```python
from build123d import *

# Parameters (mm, degrees)
SKETCH1_R             = 3.5
BOSS_EXTRUDE1_DEPTH   = 4
SKETCH2_R             = 1.925
BOSS_EXTRUDE2_DEPTH   = 10
CUT_EXTRUDE1_DEPTH    = 2
CHAMFER1_SIZE         = 0.25
CHAMFER1_SIZE2        = 0.209774908
CHAMFER1_PART_2_SIZE  = 0.25
CHAMFER1_PART_2_SIZE2 = 0.209774908
CHAMFER1_PART_3_SIZE  = 0.25
CHAMFER1_PART_3_SIZE2 = 0.209774908


with BuildPart() as part:
    # Sketch1 → Boss-Extrude1 (new body)
    with BuildSketch(Plane(origin=(0, 0, 0), x_dir=(1, 0, 0), z_dir=(0, 1, 0))):
        Circle(SKETCH1_R)
    extrude(amount=BOSS_EXTRUDE1_DEPTH)

    # Sketch2 → Boss-Extrude2 (add)
    with BuildSketch(Plane(origin=(0, 4, 0), x_dir=(1, 0, 0), z_dir=(0, 1, 0))):
        Circle(SKETCH2_R)
    extrude(amount=BOSS_EXTRUDE2_DEPTH)

    # Sketch3 → Cut-Extrude1 (cut)
    with BuildSketch(Plane.XZ):
        Polygon((0, 2.37190351), (-2.054128695, 1.185951755), (-2.054128695, -1.185951755), (0, -2.37190351), (2.054128695, -1.185951755), (2.054128695, 1.185951755), align=None)
    extrude(amount=-CUT_EXTRUDE1_DEPTH, mode=Mode.SUBTRACT)

    # Chamfer1
    chamfer1_edges = [part.edges().sort_by_distance(p)[0] for p in [
        (1.027064348, 0, 1.778927633),
        (-1.027064348, 0, 1.778927633),
        (-2.054128695, 0, 0),
        (-1.027064348, 0, -1.778927633),
        (1.027064348, 0, -1.778927633),
        (2.054128695, 0, 0),
        (-3.5, 0, 0),
    ]]
    chamfer1_side = [part.faces().sort_by_distance(p)[0] for p in [
        (-3.401005051, 0, 0),
    ]]
    chamfer(chamfer1_edges, length=CHAMFER1_SIZE, length2=CHAMFER1_SIZE2, reference=chamfer1_side[0])

    # Chamfer1 part 2
    chamfer1_part_2_edges = [part.edges().sort_by_distance(p)[0] for p in [
        (-3.5, 4, 0),
    ]]
    chamfer1_part_2_side = [part.faces().sort_by_distance(p)[0] for p in [
        (-3.5, 2, 0),
    ]]
    chamfer(chamfer1_part_2_edges, length=CHAMFER1_PART_2_SIZE, length2=CHAMFER1_PART_2_SIZE2, reference=chamfer1_part_2_side[0])

    # Chamfer1 part 3
    chamfer1_part_3_edges = [part.edges().sort_by_distance(p)[0] for p in [
        (-1.925, 14, 0),
    ]]
    chamfer1_part_3_side = [part.faces().sort_by_distance(p)[0] for p in [
        (-1.925, 9, 0),
    ]]
    chamfer(chamfer1_part_3_edges, length=CHAMFER1_PART_3_SIZE, length2=CHAMFER1_PART_3_SIZE2, reference=chamfer1_part_3_side[0])


solid = part.part
```
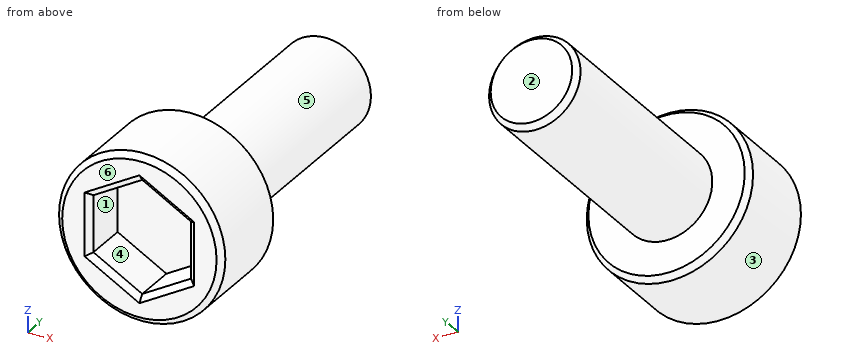
Can you work these out from the model? Positions are in its coordinate system, mm. Face numbers are marked on the shaded views. A direction names the side the tool comes from. Round coordinates to 2 decimals unless told otherwise and drop trailing zeros. Loops run counter-clockwise (first coordinate to the right, second up) from the corner with the lowest first, then second, coordinate; pieces in that order, holes last. Notation, with made-up numbers: M 13,-9 L 61,-9 A10 cw 61,5 Z; hole C 88,60 d6. An arc over 180 degrees is marked long. Answer as a JSON object with one key per item and string values. Group by question number.
Q1. Imagine slicing it at C-C, the plane y = 10.25. Please give me the cut outline in (x, z) (3 decimals), then the cut area to 3 significant figures.
Q2. Imagine slicing it at A-A, the plane z = 0. Please give me the cut outline in (x, y) (3 decimals), then the cut area to 3 significant figures.
Q3. Imagine slicing it at B-B, the plane y = 3.5. Please give me the cut outline in (x, z), then the cut area to 3 significant figures.
Q4. Please list where these lines run through material, in increasing order: L1, parallel to Y at x = -0.5, z = 0; L2, parallel to Y at x = -1, z = -3; L3, parallel to X at y = 1.5, z = 2.25.
Q5. On a 3-axis mill with a long thin cutter (end or side, diameter ignored), from which of +Z, -Z, +X, -X, +Y, -Y can I reach the whole of each face in a straight line? I mean the marked faces 4, 5 and 6. Say none if no direction works.
Q6. We'd pull the mould along X, two halves only. Please class the marked faces 1, 2 and 3: +X half, -X half, draft (parallel to the pull), parting line (faces both ways), or undercut.
Q7. Will these pins go through, and if not, where does the flat tip stop? pin 1 (0.9 mm diameter, centred on y = 1, z = -0.5, fed in from -X); pin 2 (1.5 mm diameter, centred on x = 1.5, y = 12.5, fed in from -Z); pin 3 (1 mm diameter, centred on x = -0.5, y = 7, fed in from +Z) (3 decimals).
Findings:
{
 "1": {"outline": "C 0,0 d3.85", "area": "11.6 mm2"},
 "2": {"outline": "M -3.5,0.21 L -3.25,0 L -2.304,0 L -2.054,0.21 L -2.054,2 L 2.054,2 L 2.054,0.21 L 2.304,0 L 3.25,0 L 3.5,0.21 L 3.5,3.75 L 3.29,4 L 1.925,4 L 1.925,13.75 L 1.715,14 L -1.715,14 L -1.925,13.75 L -1.925,4 L -3.29,4 L -3.5,3.75 Z", "area": "58.1 mm2"},
 "3": {"outline": "C 0,0 d7", "area": "38.5 mm2"},
 "4": {"L1": "y = 2 to 14", "L2": "y = 0 to 4", "L3": "x = -2.68 to -0.21, 0.21 to 2.68"},
 "5": {"face 4": "-Y", "face 5": "+Y", "face 6": "+Z, -Z, +X, -X, -Y"},
 "6": {"face 1": "undercut", "face 2": "draft", "face 3": "parting line"},
 "7": {"pin 1": "stops at x = -3.5", "pin 2": "stops at z = -1.77", "pin 3": "stops at z = 1.925"}
}
